CAD build for the part. Positions are in the model's coordinates, mm. Face numbers are marked on the shaded views. Give positions to 0.01 mm unless a question says otherwise; leave off trailing zeros. Order: outer loops, then holes, each group sorted by start corner. A loop starts at its lowest first (then second) coordinate and runs counter-clockwise, first axis right, second up.
Item 1: Band-saw the part on D-D on z = -57. Give the cut face in (x, y).
Item 2: Two-plate mould, pull along Y, no slides. Class the marked faces 1, 2 and 3: released by +Y, released by -Y, zero draft, split by the parting line, or undercut.
Item 3: Band-saw the part on C-C on x = 4. Give the cut face in (y, z).
Item 4: Band-saw the part on A-A on y = -13. Give the cut face in (x, z).
Item 5: Flat gauge pins, fed straight in: P1, Ø12, axis at x = 16.5, y = 12.5, coming from the -Z side; P2, Ø1.5, axis at y = -11.5, z = -34.5, coming from the +X side; P3, Ø12, axis at x = 9.5, z = -68.5, coming from the +Y side. Where does each tip first touch, or does it go through?
Item 6: Wall check: L1, parallel to X at y = -15.75, z = -80; L2, parallel to Z at x = 9.75, y = 15; L3, parallel to X at y = -4.5, z = -25.5. Give the ranges that are in metal, low to high.
Item 7: Band-saw the part on B-B on z = -21.25. Give the cut face in (x, y), plus the area to 3 significant figures.
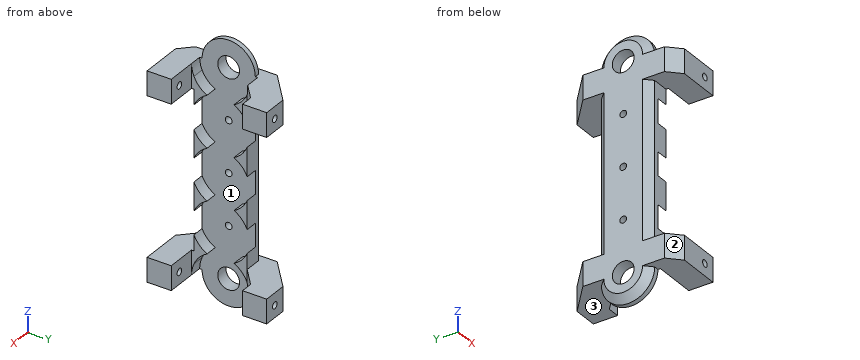
```python
from build123d import *

# Parameters (mm, degrees)
SKETCH1_R                  = 4.5
BOSS_EXTRUDE1_DEPTH        = 10
SKETCH3_R                  = 1.4
CUT_EXTRUDE1_DEPTH         = 11
BOSS_EXTRUDE2_DEPTH        = 10
LPATTERN1_COUNT            = 2
LPATTERN1_PITCH            = 75
SKETCH8_W                  = 10
SKETCH8_H                  = 10
BOSS_EXTRUDE3_DEPTH        = 1
BOSS_EXTRUDE5_START        = -10
SKETCH10_W                 = 10
SKETCH10_H                 = 10
BOSS_EXTRUDE5_DEPTH        = 22.48966
CHAMFER3_SIZE              = 5
LPATTERN3_COUNT            = 2
LPATTERN3_PITCH            = 75
CHAMFER3_OF_LPATTERN3_SIZE = 5
SKETCH6_R                  = 4.5
SKETCH6_R_2                = 1.4
SKETCH6_R_3                = 12
CUT_EXTRUDE3_DEPTH         = 10
CUT_EXTRUDE3_DEPTH_BACK    = 5
SKETCH15_R                 = 1.4
CUT_EXTRUDE4_DEPTH         = 70
CHAMFER4_SIZE              = 3


with BuildPart() as part:
    # Sketch1 → Boss-Extrude1 (new body)
    with BuildSketch(Plane(origin=(0, 0, 0), x_dir=(0, 0, -1), z_dir=(1, 0, 0))):
        with BuildLine():
            Line((0, 11), (85, 11))
            ThreePointArc((85, 11), (96, 0), (85, -11))
            Line((85, -11), (0, -11))
            ThreePointArc((0, -11), (-11, 0), (0, 11))
        make_face()
        Circle(SKETCH1_R, mode=Mode.SUBTRACT)
        with Locations((85, 0)):
            Circle(SKETCH1_R, mode=Mode.SUBTRACT)
    extrude(amount=BOSS_EXTRUDE1_DEPTH)

    # Sketch3 → Cut-Extrude1 (cut, through all)
    with BuildSketch(Plane.ZY):
        with Locations((-42.5, 0)):
            Circle(SKETCH3_R)
        with Locations((-63.75, 0)):
            Circle(SKETCH3_R)
        with Locations((-21.25, 0)):
            Circle(SKETCH3_R)
        with Locations((-148.75, 0)):
            Circle(SKETCH3_R)
        with Locations((-127.5, 0)):
            Circle(SKETCH3_R)
        with Locations((-106.25, 0)):
            Circle(SKETCH3_R)
    extrude(amount=-CUT_EXTRUDE1_DEPTH, mode=Mode.SUBTRACT)

    # Sketch8 → Boss-Extrude3 (add)
    with BuildSketch(Plane(origin=(0, -11, 0), x_dir=(-1, 0, 0), z_dir=(0, -1, 0))):
        with Locations((-5, 5)):
            Rectangle(SKETCH8_W, SKETCH8_H)
    boss_extrude3 = extrude(amount=BOSS_EXTRUDE3_DEPTH)

    # Sketch10 → Boss-Extrude5 (add)
    with BuildSketch(Plane(origin=(10, 0, 0), x_dir=(0, 0, -1), z_dir=(1, 0, 0)).offset(BOSS_EXTRUDE5_START)):
        with Locations((5, -17)):
            Rectangle(SKETCH10_W, SKETCH10_H)
    boss_extrude5 = extrude(amount=BOSS_EXTRUDE5_DEPTH)

    # Chamfer3
    chamfer3_edges = [part.edges().sort_by_distance(p)[0] for p in [
        (0, -22, -5),
    ]]
    chamfer(chamfer3_edges, length=CHAMFER3_SIZE)

    # LPattern3: Boss-Extrude3, Boss-Extrude5 ×2
    with Locations(*[(0, 0, -i * LPATTERN3_PITCH) for i in range(1, LPATTERN3_COUNT)]):
        add(boss_extrude3)
        add(boss_extrude5)

    # Chamfer3 of LPattern3
    chamfer3_of_lpattern3_edges = [part.edges().sort_by_distance(p)[0] for p in [
        (0, -22, -80),
    ]]
    chamfer(chamfer3_of_lpattern3_edges, length=CHAMFER3_OF_LPATTERN3_SIZE)


with BuildPart() as body_2:
    # Sketch7 → Boss-Extrude2 (new body)
    with BuildSketch(Plane.XY):
        Polygon((0, 11), (0, 16.697133846), (12.489660366, 27.445401219), (22.489660366, 27.445401219), (22.489660366, 17.445401219), (17.489660366, 17.445401219), (10, 11), align=None)
    boss_extrude2 = extrude(amount=-BOSS_EXTRUDE2_DEPTH)


with BuildPart() as lpattern1_1:
    # LPattern1: Boss-Extrude2 ×2
    with Locations(*[(0, 0, -i * LPATTERN1_PITCH) for i in range(1, LPATTERN1_COUNT)]):
        add(boss_extrude2)


with BuildPart() as body_2_1:
    add(body_2.part)

    # Combine1: union part, LPattern1_1
    add(part.part)
    add(lpattern1_1.part)

    # Sketch6 → Cut-Extrude3 (cut, two sides)
    with BuildSketch(Plane(origin=(10, 0, 0), x_dir=(0, 0, -1), z_dir=(1, 0, 0))) as cut_extrude3_sk:
        with BuildLine():
            ThreePointArc((10.602696958, -5.619859181), (9.250095943, -0.036989697), (10.647303042, 5.534883732))
            ThreePointArc((10.647303042, 5.534883732), (8.190816519, 8.76986458), (4.795831523, 11))
            Line((4.795831523, 11), (0, 11))
            ThreePointArc((0, 11), (-11, 0), (0, -11))
            Line((0, -11), (4.795831523, -11))
            ThreePointArc((4.795831523, -11), (8.155681986, -8.802548003), (10.602696958, -5.619859181))
        make_face()
        Circle(SKETCH6_R, mode=Mode.SUBTRACT)
        with BuildLine():
            ThreePointArc((10.647303042, 5.534883732), (11.656921474, 2.848891319), (12, 0))
            ThreePointArc((12, 0), (11.645436091, -2.895482387), (10.602696958, -5.619859181))
            ThreePointArc((10.602696958, -5.619859181), (12.983312559, -8.783359135), (16.263795125, -11))
            Line((16.263795125, -11), (26.236204875, -11))
            ThreePointArc((26.236204875, -11), (29.516687441, -8.783359135), (31.897303042, -5.619859181))
            ThreePointArc((31.897303042, -5.619859181), (30.500095943, -0.047985752), (31.852696958, 5.534883732))
            ThreePointArc((31.852696958, 5.534883732), (29.325707811, 8.791000179), (25.846011237, 11))
            Line((25.846011237, 11), (16.653988763, 11))
            ThreePointArc((16.653988763, 11), (13.174292189, 8.791000179), (10.647303042, 5.534883732))
        make_face()
        with Locations((21.25, 0)):
            Circle(SKETCH6_R_2, mode=Mode.SUBTRACT)
        Circle(SKETCH6_R_3)
        with Locations((21.25, -0.084975449)):
            Circle(SKETCH6_R_3)
        with BuildLine():
            ThreePointArc((37.704168477, 11), (34.309183481, 8.76986458), (31.852696958, 5.534883732))
            ThreePointArc((31.852696958, 5.534883732), (32.895436091, 2.810506938), (33.25, -0.084975449))
            ThreePointArc((33.25, -0.084975449), (32.906921474, -2.933866768), (31.897303042, -5.619859181))
            ThreePointArc((31.897303042, -5.619859181), (34.344318014, -8.802548003), (37.704168477, -11))
            Line((37.704168477, -11), (47.295831523, -11))
            ThreePointArc((47.295831523, -11), (50.673198678, -8.786286096), (53.125, -5.577577879))
            ThreePointArc((53.125, -5.577577879), (51.75, 0), (53.125, 5.577577879))
            ThreePointArc((53.125, 5.577577879), (50.673198678, 8.786286096), (47.295831523, 11))
            Line((47.295831523, 11), (37.704168477, 11))
        make_face()
        with Locations((42.5, 0)):
            Circle(SKETCH6_R_2, mode=Mode.SUBTRACT)
        with Locations((42.5, 0)):
            Circle(SKETCH6_R_3)
        with BuildLine():
            ThreePointArc((58.954168477, 11), (55.576801322, 8.786286096), (53.125, 5.577577879))
            ThreePointArc((53.125, 5.577577879), (54.151180198, 2.872281323), (54.5, 0))
            ThreePointArc((54.5, 0), (54.151180198, -2.872281323), (53.125, -5.577577879))
            ThreePointArc((53.125, -5.577577879), (55.576801322, -8.786286096), (58.954168477, -11))
            Line((58.954168477, -11), (68.545831523, -11))
            ThreePointArc((68.545831523, -11), (71.923198678, -8.786286096), (74.375, -5.577577879))
            ThreePointArc((74.375, -5.577577879), (73, 0), (74.375, 5.577577879))
            ThreePointArc((74.375, 5.577577879), (71.923198678, 8.786286096), (68.545831523, 11))
            Line((68.545831523, 11), (58.954168477, 11))
        make_face()
        with Locations((63.75, 0)):
            Circle(SKETCH6_R_2, mode=Mode.SUBTRACT)
        with Locations((63.75, 0)):
            Circle(SKETCH6_R_3)
        with Locations((85, 0)):
            Circle(SKETCH6_R_3)
        with BuildLine():
            ThreePointArc((80.204168477, 11), (76.826801322, 8.786286096), (74.375, 5.577577879))
            ThreePointArc((74.375, 5.577577879), (75.401180198, 2.872281323), (75.75, 0))
            ThreePointArc((75.75, 0), (75.401180198, -2.872281323), (74.375, -5.577577879))
            ThreePointArc((74.375, -5.577577879), (76.826801322, -8.786286096), (80.204168477, -11))
            Line((80.204168477, -11), (85, -11))
            ThreePointArc((85, -11), (96, 0), (85, 11))
            Line((85, 11), (80.204168477, 11))
        make_face()
        with Locations((85, 0)):
            Circle(SKETCH6_R, mode=Mode.SUBTRACT)
        with BuildLine():
            Line((0, 11), (4.795831523, 11))
            ThreePointArc((4.795831523, 11), (-12, 0), (4.795831523, -11))
            Line((4.795831523, -11), (0, -11))
            ThreePointArc((0, -11), (-11, 0), (0, 11))
        make_face()
        with BuildLine():
            ThreePointArc((97, 0), (91.574573055, 10.03867467), (80.204168477, 11))
            Line((80.204168477, 11), (85, 11))
            ThreePointArc((85, 11), (96, 0), (85, -11))
            Line((85, -11), (80.204168477, -11))
            ThreePointArc((80.204168477, -11), (91.574573055, -10.03867467), (97, 0))
        make_face()
    extrude(amount=CUT_EXTRUDE3_DEPTH, mode=Mode.SUBTRACT)
    extrude(cut_extrude3_sk.sketch, amount=-CUT_EXTRUDE3_DEPTH_BACK, mode=Mode.SUBTRACT)

    # Sketch15 → Cut-Extrude4 (cut)
    with BuildSketch(Plane(origin=(0, 27.445401219, 0), x_dir=(1, 0, 0), z_dir=(0, 1, 0))):
        with Locations((17.489660366, 80)):
            Circle(SKETCH15_R)
        with Locations((17.489660366, 5)):
            Circle(SKETCH15_R)
    extrude(amount=-CUT_EXTRUDE4_DEPTH, mode=Mode.SUBTRACT)

    # Chamfer4
    chamfer4_edges = [body_2_1.edges().sort_by_distance(p)[0] for p in [
        (0, -11, -42.5),
        (0, 11, -42.5),
        (0, 0, -96),
        (0, 0, 11),
    ]]
    chamfer(chamfer4_edges, length=CHAMFER4_SIZE)


solid = body_2_1.part
```
The answers:
1. outline: (0, -8) - (3, -11) - (10, -11) - (10, -9.92) - (5, -9.92) - (5, 9.92) - (10, 9.92) - (10, 11) - (3, 11) - (0, 8) - close
2. face 1: undercut
2. face 2: released by -Y
2. face 3: zero draft
3. outline: (-21, -85) - (-11, -85) arc R11 ccw to (11, -85) - (20.14, -85) - (20.14, -75) - (11, -75) - (11, -10) - (20.14, -10) - (20.14, 0) - (11, 0) arc R11 ccw to (-11, 0) - (-21, 0) - (-21, -10) - (-11, -10) - (-11, -75) - (-21, -75) - close; hole circle Ø9 at (0, -85); hole circle Ø9 at (0, 0); hole circle Ø2.8 at (0, -63.75); hole circle Ø2.8 at (0, -42.5); hole circle Ø2.8 at (0, -21.25)
4. outline: (0, -85) - (22.49, -85) - (22.49, -75) - (0, -75) - close; (0, -10) - (22.49, -10) - (22.49, 0) - (0, 0) - close; hole circle Ø2.8 at (17.49, -80); hole circle Ø2.8 at (17.49, -5)
5. P1: stops at z = -85
5. P2: stops at x = 10
5. P3: stops at y = 11
6. L1: x = 0 to 16.09, 18.89 to 22.49
6. L2: z = -85 to -75, -10 to 0
6. L3: x = 0 to 5
7. outline: (0, -8) - (3, -11) - (5, -11) - (5, -1.4) - (0, -1.4) - close; (0, 1.4) - (5, 1.4) - (5, 11) - (3, 11) - (0, 8) - close
7. area: 87.0 mm2
